```python
from build123d import *

# Parameters (mm, degrees)
F0_R     = 13.0048
F1_DEPTH = 20.0025
F2_DEPTH = 5.9944
F0_R_2   = 5.9944
F3_DEPTH = 13.0048


with BuildPart() as f1:
    # F0 (on Front) → F1 (new body, symmetric)
    with BuildSketch(Plane.XZ):
        with BuildLine():
            ThreePointArc((-12.949346, -21.392276), (12.278025, -21.784516), (25.0063, 0))
            ThreePointArc((25.0063, 0), (13.562501, 21.008894), (-10.294693, 22.788908))
            ThreePointArc((-10.294693, 22.788908), (-24.961282, 1.499814), (-12.949346, -21.392276))
        make_face()
        Circle(F0_R, mode=Mode.SUBTRACT)
    extrude(amount=F1_DEPTH, both=True)

    # F0 (on Front) → F2 (join, symmetric)
    with BuildSketch(Plane.XZ):
        with BuildLine():
            ThreePointArc((-12.949346, -21.392276), (-24.961282, 1.499814), (-10.294693, 22.788908))
            Line((-10.294693, 22.788908), (-102.934025, -19.060113))
            ThreePointArc((-102.934025, -19.060113), (-91.484026, -19.914411), (-85.9917, -29.9974))
            ThreePointArc((-85.9917, -29.9974), (-97.9932, -41.9989), (-109.9947, -29.9974))
            Line((-109.9947, -29.9974), (-109.9947, -70.0024))
            ThreePointArc((-109.9947, -70.0024), (-97.9932, -58.0009), (-85.9917, -70.0024))
            ThreePointArc((-85.9917, -70.0024), (-87.042616, -74.913685), (-90.011317, -78.964852))
            Line((-90.011317, -78.964852), (-25.365987, -21.392276))
            ThreePointArc((-25.365987, -21.392276), (-19.157667, -19.6596), (-12.949346, -21.392276))
        make_face()
    extrude(amount=F2_DEPTH, both=True)

    # F0 (on Front) → F3 (join, symmetric)
    with BuildSketch(Plane.XZ):
        with BuildLine():
            ThreePointArc((-85.9917, -29.9974), (-91.484026, -19.914411), (-102.934025, -19.060113))
            ThreePointArc((-102.934025, -19.060113), (-108.076189, -23.488226), (-109.9947, -29.9974))
            ThreePointArc((-109.9947, -29.9974), (-97.9932, -41.9989), (-85.9917, -29.9974))
        make_face()
        with Locations((-97.9932, -29.9974)):
            Circle(F0_R_2, mode=Mode.SUBTRACT)
        with BuildLine():
            ThreePointArc((-109.9947, -70.0024), (-102.904485, -80.952984), (-90.011317, -78.964852))
            ThreePointArc((-90.011317, -78.964852), (-87.042616, -74.913685), (-85.9917, -70.0024))
            ThreePointArc((-85.9917, -70.0024), (-97.9932, -58.0009), (-109.9947, -70.0024))
        make_face()
        with Locations((-97.9932, -70.0024)):
            Circle(F0_R_2, mode=Mode.SUBTRACT)
    extrude(amount=F3_DEPTH, both=True)


solid = f1.part
```
Can you work these out from the model? Positions are in its coordinate system, mm. A direction names the side the tool comes from. Give positions to 0.01 mm unless a question says otherwise; leave off trailing zeros. Loops run counter-clockwise (first coordinate to the right, second up) from the corner with the lowest first, then second, coordinate; pieces in that order, holes last. Notation, with made-up numbers: M 52.25,24 L 56.25,24 A22 cw 56.25,58 Z; hole C -36,80.25 d8. An arc over 180 degrees is marked long. Use one line per item in the form item = value. Start each with the question number.
(1) I want a section at D-D, the plane y = 17. Write out the boundary of the cut face in (x, z).
(2) Thinking about a two-plate mould opening in X: for faces 1 (the flat face through (-55.966, -0.084, 2.157)), 2 (the flat face through (-95, 13.005, -24)), 3 (the cylindrical face through (-103.98, 0.18, -29.73)), which applies, released by +X, released by -X, zero draft, split by the parting line, or undercut?
(3) I want a section at A-A, the plane y = 10. Write out the boundary of the cut face in (x, z).
(4) I'm going to push flat-ended pins straight in: P1, Ø12, axis at x = -97.5, z = -31.5, coming from the -Y side; P2, Ø3, axis at y = -3, z = -26.5, coming from the -X side; P3, Ø1, axis at x = -58, y = 4.5, coming from the +Z side; P4, Ø9.5, axis at x = -97.99, z = -70, coming from the -Y side. Where does each tip first touch, or does it pass through?
(5) I want a section at B-B, the plane x = 0. Write out the boundary of the cut face in (y, z), and give its area (3 significant figures).
(6) Please list where these lines run through material, in increasing order: line 1 (X direction, y = -10.5, z = -0.5); line 2 (Z direction, x = 0, y = -5.5); line 3 (Z direction, x = -102, y = 11).
(7) On a 3-axis mill with a long thin cutter (end or side, diameter ignored), from which of +Z, -Z, +X, -X, +Y, -Y can I reach the whole of each face in a straight line? I mean faces 4 (the flat face through (-95, -13.005, -24)), 5 (the flat face through (11, 20.002, -11)). Say none if no direction works.
(8) I want a section at C-C, the plane z = -68.5. Write out the boundary of the cut face in (x, y).
Worked out:
q1.outline = C 0,0 d50.01; hole C 0,0 d26.01
q2.face_1 = released by -X
q2.face_2 = zero draft
q2.face_3 = undercut
q3.outline = M -109.99,-30 A12 ccw long -102.93,-19.06 A12 ccw Z; M -90.01,-78.96 A12 ccw -85.99,-70 A12 ccw long Z; C 0,0 d50.01; hole C -97.99,-70 d11.99; hole C -97.99,-30 d11.99; hole C 0,0 d26.01
q4.P1 = -13
q4.P2 = -109.83
q4.P3 = 1.46
q4.P4 = through
q5.outline = M -20,-25.01 L 20,-25.01 L 20,-13 L -20,-13 Z; M -20,13 L 20,13 L 20,25.01 L -20,25.01 Z
q5.area = 960 mm²
q6.line_1 = -25 to -13, 13 to 25
q6.line_2 = -25.01 to -13, 13 to 25.01
q6.line_3 = -81.32 to -74.46, -65.54 to -58.69, -41.31 to -34.46, -25.54 to -18.68
q7.face_4 = +Z, -Z, -X, -Y
q7.face_5 = +Z, -Z, +X, -X, +Y
q8.outline = M -109.99,-5.99 L -109.9,-5.99 L -109.9,-13 L -103.8,-13 L -103.8,13 L -109.9,13 L -109.9,5.99 L -109.99,5.99 Z; M -92.19,-13 L -86.09,-13 L -86.09,-5.99 L -78.26,-5.99 L -78.26,5.99 L -86.09,5.99 L -86.09,13 L -92.19,13 Z
